The model under review builds one solid part; all positions refer to its coordinate system, in mm. A direction names the side the tool comes from. Round coordinates to 2 decimals unless told otherwise and drop trailing zeros. Write each loop counter-clockwise with the first axis right and the second up, starting at its lowest first coordinate (ties: lowest second). Pieces come first, ordered by that corner, then holes. Notation, with made-up numbers: (44, -33.5) - (58, -33.5) arc R17 ccw to (58, -22.5) - close; hole circle Ø9 at (87, 2). An arc over 180 degrees is marked (long way). Write each question's results on one line, items separated by ' | '.
```python
from build123d import *

# Parameters (mm, degrees)
BOSS_EXTRUDE1_DEPTH = 30.48
SKETCH2_R           = 2.3495
CUT_EXTRUDE1_DEPTH  = 10
BOSS_EXTRUDE2_START = 14.99
BOSS_EXTRUDE2_DEPTH = 0.5


with BuildPart() as part:
    # Sketch1 → Boss-Extrude1 (new body)
    with BuildSketch(Plane(origin=(0, 0, 0), x_dir=(0, 0, -1), z_dir=(1, 0, 0))):
        Polygon((10.247, -6.144), (10.247, 0), (0, 0), (0, -2.794), (7.747, -2.794), (7.747, -9.144), (27.432, -9.144), (27.432, 0), (22.432, 0), (16.247, -6.144), align=None)
    extrude(amount=BOSS_EXTRUDE1_DEPTH)

    # Sketch2 → Cut-Extrude1 (cut)
    with BuildSketch(Plane(origin=(0, 0, 0), x_dir=(1, 0, 0), z_dir=(0, 1, 0))):
        with Locations(Location((5.08, 3.937, 0), (0, 0, 270))):
            Circle(SKETCH2_R)
        with Locations(Location((15.24, 3.937, 0), (0, 0, 270))):
            Circle(SKETCH2_R)
        with Locations(Location((25.4, 3.937, 0), (0, 0, 270))):
            Circle(SKETCH2_R)
        Polygon((9, 27.432), (0, 10.247), (0, 27.432), align=None)
        Polygon((21.48, 27.432), (30.48, 10.247), (30.48, 27.432), align=None)
    extrude(amount=-CUT_EXTRUDE1_DEPTH, mode=Mode.SUBTRACT)

    # Sketch1_4 → Boss-Extrude2 (add)
    with BuildSketch(Plane(origin=(0, 0, 0), x_dir=(0, 0, -1), z_dir=(1, 0, 0)).offset(BOSS_EXTRUDE2_START)):
        Polygon((34.29, -21.59), (35.29, -21.59), (35.814, -22.114), (35.814, -23.114), align=None)
        Polygon((27.432, -8.144), (27.432, -9.144), (34.29, -9.144), (34.29, -21.59), (35.29, -21.59), (35.29, -8.144), align=None)
    extrude(amount=BOSS_EXTRUDE2_DEPTH)


solid = part.part
```
Q1. We need section B-B (x = 21). State the section outline as (y, z) points, plus the area to 3 significant figures.
Evaluation:
outline: (-9.14, -27.43) - (0, -27.43) - (0, -22.43) - (-6.14, -16.25) - (-6.14, -10.25) - (0, -10.25) - (0, 0) - (-2.79, 0) - (-2.79, -7.75) - (-9.14, -7.75) - close | area: 146 mm^2
Q2. For probe 1 along Y at (x, z) = (16, -13); probe 2 along Y at (x, z) = (14, -24); probe 3 along Z at (x, y) = (24, -4.5), list the stretches that pass through material, from the lowest coordinate up.
Evaluation:
probe 1: y = -9.14 to -6.14 | probe 2: y = -9.14 to 0 | probe 3: z = -22.62 to -17.9, -10.25 to -7.75
Q3. We need section A-A (x = 4). State the section outline as (y, z) points, plus the area to 3 significant figures.
Evaluation:
outline: (-9.14, -17.88) - (-4.52, -17.88) - (-6.14, -16.25) - (-6.14, -10.25) - (0, -10.25) - (0, -6.02) - (-2.79, -6.02) - (-2.79, -7.75) - (-9.14, -7.75) - close; (-2.79, -1.85) - (0, -1.85) - (0, 0) - (-2.79, 0) - close | area: 57.1 mm^2
Q4. Tool access review of faces 4 (the flat face through (15, -6, -7.747)), 5 (the flat face through (5.563, -5.524, -20.869)), 6 (the flat face through (0, -2, -6)), 7 (the flat face through (15, -3, -10.247)), 8 (the flat face through (15.49, -13, -35)): name each direction out of +Z, -Z, +X, -X, +Y, -Y from which nothing blocks a thin tool from reaching the whole face with its end or side.
Evaluation:
face 4: +Z, +X, -X, -Y | face 5: -Z, -X, +Y, -Y | face 6: +Z, -Z, -X, +Y, -Y | face 7: +X, -X, +Y | face 8: -Z, +X, +Y, -Y
Q5. We need section C-C (y = -4). State the section outline as (x, z) points, plus the area to 3 significant figures.
Evaluation:
outline: (0, -10.25) - (30.48, -10.25) - (30.48, -7.75) - (0, -7.75) - close; (4.27, -18.41) - (9, -27.43) - (21.48, -27.43) - (26.21, -18.41) - close | area: 232 mm^2
Q6. Insertion check: P1, Ø3, axis at x = 19, z = -12.5, coming from the +Y side; P2, Ø2, axis at x = 19, z = -11, coming from the -Y side; P3, Ø5, axis at x = 16.5, y = -6, coming from the +Z side; P4, Ø6, axis at x = 17.5, z = -21, coming from the +Y side. Each pin has a flat end and moves straight along its axis. Give the tip position at first contact, or say it passes through.
Evaluation:
P1: stops at y = -6.14 | P2: stops at y = -9.14 | P3: stops at z = -7.75 | P4: stops at y = 0
Q7. We need section D-D (x = 14). State the section outline as (y, z) points.
Evaluation:
outline: (-9.14, -27.43) - (0, -27.43) - (0, -22.43) - (-6.14, -16.25) - (-6.14, -10.25) - (0, -10.25) - (0, -5.93) - (-2.79, -5.93) - (-2.79, -7.75) - (-9.14, -7.75) - close; (-2.79, -1.94) - (0, -1.94) - (0, 0) - (-2.79, 0) - close
Q8. The part is to be moulded in two halves that separate along Z. For faces 1 (the flat face through (15, -6.144, -13)), 2 (the flat face through (30.48, -2, -6)), 3 (the flat face through (15.2, -22.4, -35.1)), say which applies: released by +Z, released by -Z, zero draft, split by the parting line, or undercut.
Evaluation:
face 1: undercut | face 2: zero draft | face 3: released by +Z
